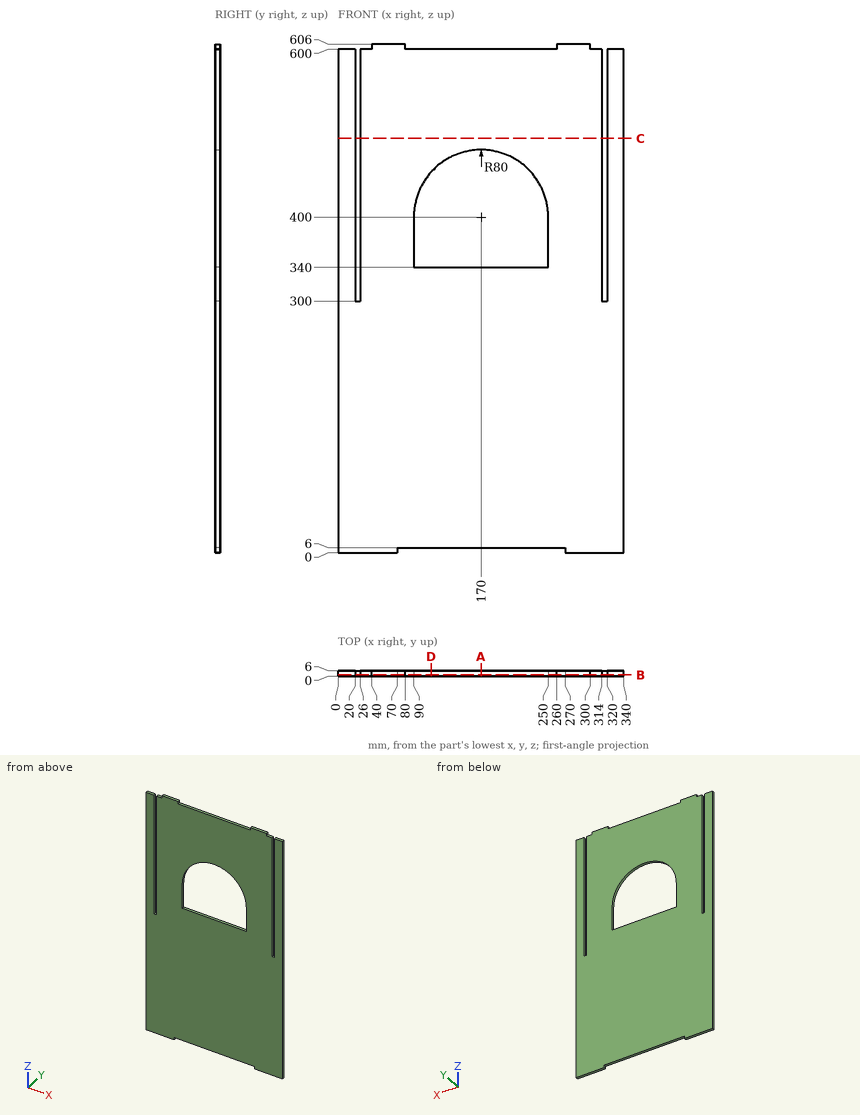
Study the drawing (mm; zero at the part's minimum x, y, z) and answer. Coordinates: 2 decimals unless noted, no trailing zeros. Order: outer loops, then holes, each group sorted by start corner. A loop starts at its lowest first (then second) coordinate and runs counter-clockwise, first axis right, second up. Notation, with made-up numbers: M 67,40 L 77,40 A5 ccw 77,46 Z; hole C 3,71 d11. An arc over 180 degrees is marked long. Use CSV: the item, a comma, the result in double quotes.
Q1. Section A-A (x = 170) is taken. Determine the outline of the cut face in (y, z), then the cut area to 3 significant figures.
Here are the results:
outline,"M 0,6 L 6,6 L 6,340 L 0,340 Z; M 0,480 L 6,480 L 6,600 L 0,600 Z"
area,"2,720 mm2"
Q2. Given pin 1 Ø3 at (y, z) = (3, 604) entering from +X; pin 2 Ø1 at (x, y) = (254, 4.5) entering from +Z, each flat-ended and moving along its own axis, determine where each tip first touches the part or whether it passes through.
Here are the results:
pin 1,"x = 300"
pin 2,"z = 600"
Q3. Straight lines are drawn through the part: L1, parallel to X at y = 4.9, z = 401.5; L2, parallel to X at y = 4.3, z = 556; L3, parallel to X at y = 3, z = 414. For each, find the intervals that lie inside material, in ascending order.
Here are the results:
L1,"0 to 20, 26 to 90.01, 249.99 to 314, 320 to 340"
L2,"0 to 20, 26 to 314, 320 to 340"
L3,"0 to 20, 26 to 91.23, 248.77 to 314, 320 to 340"
Q4. Section D-D (x = 110.5) is taken. Determine the outline of the cut face in (y, z).
Here are the results:
outline,"M 0,6 L 6,6 L 6,340 L 0,340 Z; M 0,453.48 L 6,453.48 L 6,600 L 0,600 Z"
Q5. Section B-B (y = 1.2) is taken. Determine the outline of the cut face in (x, z), then the cut area to 3 significant figures.
Here are the results:
outline,"M 0,0 L 70,0 L 70,6 L 270,6 L 270,0 L 340,0 L 340,600 L 320,600 L 320,300 L 314,300 L 314,600 L 300,600 L 300,606 L 260,606 L 260,600 L 80,600 L 80,606 L 40,606 L 40,600 L 26,600 L 26,300 L 20,300 L 20,600 L 0,600 Z; hole M 90,340 L 250,340 L 250,400 A80 ccw 90,400 Z"
area,"180,000 mm2"
Q6. Section C-C (z = 493.5) is taken. Determine the outline of the cut face in (x, y).
Here are the results:
outline,"M 0,0 L 20,0 L 20,6 L 0,6 Z; M 26,0 L 314,0 L 314,6 L 26,6 Z; M 320,0 L 340,0 L 340,6 L 320,6 Z"
